The listing builds one solid part. Answer for the finished solid, in the listing's coordinates (mm). Round coordinates to 2 decimals unless told otherwise and drop trailing zeros. Write each loop counter-clockwise with the first axis right and the second up, starting at its lowest first coordinate (ties: lowest second). Pieces come first, ordered by that corner, then holes. Notation, with made-up numbers: M 82.25,-14.5 L 112.25,-14.5 A11 ccw 112.25,-4.5 Z; hole C 17.5,30.5 d6. An arc over 180 degrees is marked long. Put each result on its own line as item: value. Start each with the question number.
Autodesk Inventor part; units mm, degrees
ref_plane "YZ Plane" through (0, 0, 0) normal (1, 0, 0) x (0, 1, 0)
ref_plane "XZ Plane" through (0, 0, 0) normal (0, 1, 0) x (-1, 0, 0)
ref_plane "XY Plane" through (0, 0, 0) normal (0, 0, 1) x (1, 0, 0)
sketch "Sketch1" plane through (0, 0, 0) normal (0, 0, 1) x (1, 0, 0)
  line L0 (-25, 7.5) -> (25, 7.5)
  line L1 (25, 7.5) -> (25, -7.5)
  line L2 (25, -7.5) -> (-25, -7.5)
  line L3 (-25, -7.5) -> (-25, 7.5)
  line L4 (0, 0) -> (0, 14.2686)
  line L5 (0, 0) -> (7.5147, 0)
  dimension "d2" = 50
  dimension "d3" = 15
extrude "Extrusion1" add sketch "Sketch1" along normal blind 1000
sketch "Sketch4" plane through (-25, 7.5, 0) normal (0, 1, 0) x (1, 0, 0)
  line L0 (25, 0) -> (25, -1000)
  line L1 (0, -1000) -> (50, -1000)
  line L2 (0, 0) -> (0, -1000)
  line L3 (0, -500) -> (50, -500)
  line L4 (50, 0) -> (50, -1000)
  line L5 (25, -530) -> (10, -530)
  line L6 (10, -530) -> (10, -470)
  line L7 (10, -470) -> (25, -470)
  line L8 (25, -470) -> (25, -530)
  dimension "d14" = 15
  dimension "d15" = 60
extrude "Extrusion4" cut sketch "Sketch4" against normal through all contours L5 L6 L3 L0 | L3 L6 L7 L0
sketch "Sketch5" plane through (0, 7.5, 470) normal (-1, 0, 0) x (0, 0, 1)
  line L0 (0, 0) -> (60, 0)
  line L1 (30, 0) -> (30, -15)
  line L2 (60, -15) -> (0, -15)
  line L3 (60, 0) -> (60, -15)
  line L4 (60, -7.5) -> (0, -7.5)
  line L5 (0, 0) -> (0, -15)
  circle A0 centre (30, -7.5) radius 5
  point P0 (-470, -7.5)
  dimension "d18" = 10
extrude "Extrusion5" cut sketch "Sketch5" along normal through all both and the other way through all contours A0 L4 L1 | L1 L4 A0 | L4 L1 A0 | L4 A0 L1
properties part number "Layer"
Item 1: Section A-A (y = 0) is taken. Give the vertices of the cut face in (x, z), and give its area (4 significant figures).
Item 2: A flat-ended cylindrical pin translates along its axis: pin 1 (9 mm diameter, centred on y = 0, z = 500, fed in from +X). Find the tip coordinate at first contact, or state that the pin passes through.
Item 3: Determine the mould class of faces 1 (the flat face through (5, 7.5, 493)), 2 (the flat face through (0.3, -7.5, 493)) for opening direction Y: released by +Y, released by -Y, zero draft, split by the parting line, or undercut.
Item 4: Consider line 1 along Z through (x, y) = (-16.75, 0); line 2 along Z through (x, y) = (-7.5, -6.75); line 3 along Y through (x, z) = (-20.75, 500). Determine where each line is inside the solid, lowest interval first. Write a range as [from, to].
Output values:
1. outline: M -25,0 L 25,0 L 25,495 L 0,495 L 0,470 L -15,470 L -15,495 L -25,495 Z; M -25,505 L -15,505 L -15,530 L 0,530 L 0,505 L 25,505 L 25,1000 L -25,1000 Z
1. area: 48,750 mm^2
2. pin 1: passes through
3. face 1: released by +Y
3. face 2: released by -Y
4. line 1: z = [0, 495], [505, 1000]
4. line 2: z = [0, 470], [530, 1000]
4. line 3: y = [-7.5, -5], [5, 7.5]
